Could you check a few things on this model? Use its own coordinates, in mm. Face numbers are marked on the shaded views. A direction names the side the tool comes from. Give positions to 0.01 mm unless a question says otherwise; leave off trailing zeros. Loops run counter-clockwise (first coordinate to the right, second up) from the corner with the lowest first, then second, coordinate; pieces in that order, holes last. Notation, with made-up numbers: M -26,9.5 L 25,9.5 A26 cw 25,36.5 Z; hole C 50.25,63.5 d11. An arc over 180 degrees is marked long. Return JSON: item names as keys, results as strings. Group by question number.
1. If we section it at B-B (z = 83.5): Write out the boundary of the cut face in (x, y).
2. For pin 1 (10 mm diameter, centred on x = 73, y = 48.5, fed in from +Z); pin 2 (8 mm diameter, centred on y = -6, z = 58.5, fed in from +X); pin 3 (5 mm diameter, centred on x = 53, y = 39.5, fed in from -Z); pin 4 (22 mm diameter, centred on x = 213.5, z = -4, fed in from +Y), each with a flat end and sliding along its axis, tell me the tip position at first contact or that it passes through.
3. For the marked faces 1 and 2, which set-ups out of +Z, -Z, +X, -X, +Y, -Y let a thin tool reach every point of the face, with its end or its side?
4. If we mould it in two halves opening along Z, with no side actions, what happens to the marked faces 3, 4 and 5? For each: +Z half, -Z half, draft (parallel to the pull), parting line (faces both ways), or undercut.
5. If we section it at A-A (x = 120): Write out the boundary of the cut face in (y, z).
6. If we section it at C-C (y = 53): Write out the boundary of the cut face in (x, z).
7. If we section it at D-D (x = 59.5): Write out the boundary of the cut face in (y, z).
8. Please list where these lines run through material, in increasing order: line 1 (X direction, y = 59, z = 70); line 2 (Z direction, x = 142.5, y = 12.5); line 3 (Z direction, x = 215, y = 66.05).
```python
from build123d import *

# Parameters (mm, degrees)
SKETCH1_W           = 200
SKETCH1_H           = 125
BOSS_EXTRUDE1_DEPTH = 70
SKETCH2_W           = 210
SKETCH2_H           = 135
BOSS_EXTRUDE2_DEPTH = 10
SKETCH3_R           = 10
BOSS_EXTRUDE5_DEPTH = 5
CUT_EXTRUDE2_DEPTH  = 5
CUT_EXTRUDE3_DEPTH  = 10
SKETCH10_W          = 10
SKETCH10_H          = 125
CUT_EXTRUDE4_DEPTH  = 10
BOSS_EXTRUDE6_DEPTH = 5
SKETCH12_R          = 8
CUT_EXTRUDE5_DEPTH  = 10


with BuildPart() as part:
    # Sketch1 → Boss-Extrude1 (new body)
    with BuildSketch(Plane(origin=(0, 0, 0), x_dir=(1, 0, 0), z_dir=(0, 1, 0))):
        Polygon((210, 0), (0, 0), (0, -135), (5, -135), (210, -135), align=None)
        with Locations((105, -67.5)):
            Rectangle(SKETCH1_W, SKETCH1_H, mode=Mode.SUBTRACT)
    extrude(amount=BOSS_EXTRUDE1_DEPTH)

    # Sketch2 → Boss-Extrude2 (add)
    with BuildSketch(Plane(origin=(0, 0, 0), x_dir=(-1, 0, 0), z_dir=(0, -1, 0))):
        with Locations((-105, -67.5)):
            Rectangle(SKETCH2_W, SKETCH2_H)
    extrude(amount=BOSS_EXTRUDE2_DEPTH)

    # Sketch3 → Boss-Extrude5 (add)
    with BuildSketch(Plane(origin=(0, -10, 0), x_dir=(-1, 0, 0), z_dir=(0, -1, 0))):
        with Locations((-210, 0)):
            Circle(SKETCH3_R)
        Circle(SKETCH3_R)
        with Locations((0, -135)):
            Circle(SKETCH3_R)
        with Locations((-210, -135)):
            Circle(SKETCH3_R)
    extrude(amount=-BOSS_EXTRUDE5_DEPTH)

    # Sketch7 → Cut-Extrude2 (cut)
    with BuildSketch(Plane(origin=(0, -5, 0), x_dir=(1, 0, 0), z_dir=(0, 1, 0))):
        with BuildLine():
            ThreePointArc((215.235533906, -138.535533906), (214.186095741, -136.964938701), (212.333452378, -137.333452378))
            Line((212.333452378, -137.333452378), (214.737615434, -139.737615434))
            ThreePointArc((214.737615434, -139.737615434), (215.106129111, -139.186095741), (215.235533906, -138.535533906))
        make_face()
        with BuildLine():
            Line((214.737615434, -139.737615434), (212.333452378, -137.333452378))
            ThreePointArc((212.333452378, -137.333452378), (212.333452378, -139.737615434), (214.737615434, -139.737615434))
        make_face()
        with BuildLine():
            ThreePointArc((214.737615434, 4.737615434), (212.333452378, 4.737615434), (212.333452378, 2.333452378))
            Line((212.333452378, 2.333452378), (214.737615434, 4.737615434))
        make_face()
        with BuildLine():
            Line((214.737615434, 4.737615434), (212.333452378, 2.333452378))
            ThreePointArc((212.333452378, 2.333452378), (214.186095741, 1.964938701), (215.235533906, 3.535533906))
            ThreePointArc((215.235533906, 3.535533906), (215.106129111, 4.186095741), (214.737615434, 4.737615434))
        make_face()
        with BuildLine():
            ThreePointArc((-4.737615434, 4.737615434), (-4.737615434, 2.333452378), (-2.333452378, 2.333452378))
            Line((-2.333452378, 2.333452378), (-4.737615434, 4.737615434))
        make_face()
        with BuildLine():
            Line((-4.737615434, 4.737615434), (-2.333452378, 2.333452378))
            ThreePointArc((-2.333452378, 2.333452378), (-1.964938701, 2.884972071), (-1.835533906, 3.535533906))
            ThreePointArc((-1.835533906, 3.535533906), (-2.884972071, 5.106129111), (-4.737615434, 4.737615434))
        make_face()
        with BuildLine():
            ThreePointArc((-1.835533906, -138.535533906), (-1.964938701, -137.884972071), (-2.333452378, -137.333452378))
            Line((-2.333452378, -137.333452378), (-4.737615434, -139.737615434))
            ThreePointArc((-4.737615434, -139.737615434), (-2.884972071, -140.106129111), (-1.835533906, -138.535533906))
        make_face()
        with BuildLine():
            Line((-4.737615434, -139.737615434), (-2.333452378, -137.333452378))
            ThreePointArc((-2.333452378, -137.333452378), (-4.737615434, -137.333452378), (-4.737615434, -139.737615434))
        make_face()
    extrude(amount=-CUT_EXTRUDE2_DEPTH, mode=Mode.SUBTRACT)

    # Sketch9 → Cut-Extrude3 (cut)
    with BuildSketch(Plane(origin=(0, 0, 0), x_dir=(1, 0, 0), z_dir=(0, 1, 0))):
        Polygon((195, -130), (200, -125), (205, -120), (205, -15), (200, -10), (195, -5), align=None)
    extrude(amount=-CUT_EXTRUDE3_DEPTH, mode=Mode.SUBTRACT)

    # Sketch10 → Cut-Extrude4 (cut)
    with BuildSketch(Plane(origin=(0, 0, 0), x_dir=(1, 0, 0), z_dir=(0, 1, 0))):
        with Locations((190, -67.5)):
            Rectangle(SKETCH10_W, SKETCH10_H)
    extrude(amount=-CUT_EXTRUDE4_DEPTH, mode=Mode.SUBTRACT)

    # Sketch11 → Boss-Extrude6 (add)
    with BuildSketch(Plane(origin=(0, 70, 0), x_dir=(1, 0, 0), z_dir=(0, 1, 0))):
        with BuildLine():
            ThreePointArc((213.3, -67.5), (215, -65.8), (216.7, -67.5))
            Line((216.7, -67.5), (220, -67.5))
            ThreePointArc((220, -67.5), (217.071067812, -60.428932188), (210, -57.5))
            Line((210, -57.5), (210, -67.5))
            Line((210, -67.5), (213.3, -67.5))
        make_face()
        with BuildLine():
            Line((220, -67.5), (216.7, -67.5))
            ThreePointArc((216.7, -67.5), (215, -69.2), (213.3, -67.5))
            Line((213.3, -67.5), (210, -67.5))
            Line((210, -67.5), (210, -77.5))
            ThreePointArc((210, -77.5), (217.071067812, -74.571067812), (220, -67.5))
        make_face()
        with BuildLine():
            Line((205, -76.160254038), (205, -58.839745962))
            ThreePointArc((205, -58.839745962), (200, -67.5), (205, -76.160254038))
        make_face()
        with BuildLine():
            Line((210, -67.5), (210, -57.5))
            ThreePointArc((210, -57.5), (207.411809549, -57.840741737), (205, -58.839745962))
            Line((205, -58.839745962), (205, -76.160254038))
            ThreePointArc((205, -76.160254038), (207.411809549, -77.159258263), (210, -77.5))
            Line((210, -77.5), (210, -67.5))
        make_face()
        with BuildLine():
            ThreePointArc((10, -67.5), (8.660254038, -62.5), (5, -58.839745962))
            Line((5, -58.839745962), (5, -76.160254038))
            ThreePointArc((5, -76.160254038), (8.660254038, -72.5), (10, -67.5))
        make_face()
        with BuildLine():
            Line((0, -57.5), (0, -67.5))
            Line((0, -67.5), (0, -77.5))
            ThreePointArc((0, -77.5), (2.588190451, -77.159258263), (5, -76.160254038))
            Line((5, -76.160254038), (5, -58.839745962))
            ThreePointArc((5, -58.839745962), (2.588190451, -57.840741737), (0, -57.5))
        make_face()
        with BuildLine():
            Line((0, -77.5), (0, -67.5))
            Line((0, -67.5), (-3.3, -67.5))
            ThreePointArc((-3.3, -67.5), (-5, -69.2), (-6.7, -67.5))
            Line((-6.7, -67.5), (-10, -67.5))
            ThreePointArc((-10, -67.5), (-7.071067812, -74.571067812), (0, -77.5))
        make_face()
        with BuildLine():
            Line((-3.3, -67.5), (0, -67.5))
            Line((0, -67.5), (0, -57.5))
            ThreePointArc((0, -57.5), (-7.071067812, -60.428932188), (-10, -67.5))
            Line((-10, -67.5), (-6.7, -67.5))
            ThreePointArc((-6.7, -67.5), (-5, -65.8), (-3.3, -67.5))
        make_face()
    extrude(amount=-BOSS_EXTRUDE6_DEPTH)

    # Sketch12 → Cut-Extrude5 (cut)
    with BuildSketch(Plane(origin=(0, 0, 0), x_dir=(-1, 0, 0), z_dir=(0, 0, -1))):
        with Locations((-75, 17.5)):
            Circle(SKETCH12_R)
        with Locations((-120, 20)):
            Circle(SKETCH12_R)
    extrude(amount=-CUT_EXTRUDE5_DEPTH, mode=Mode.SUBTRACT)


solid = part.part
```
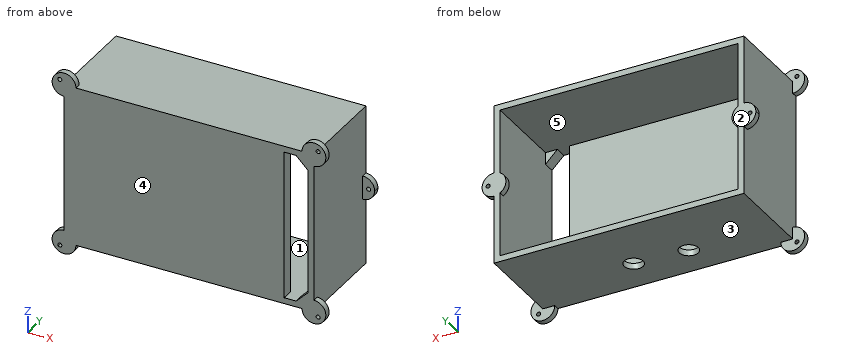
Answer:
{
 "1": {"outline": "M 0,-10 L 185,-10 L 185,0 L 5,0 L 5,70 L 0,70 Z; M 205,-10 L 210,-10 L 210,70 L 205,70 Z"},
 "2": {"pin 1": "stops at z = 135", "pin 2": "stops at x = 210", "pin 3": "stops at z = 0", "pin 4": "stops at y = 70"},
 "3": {"face 1": "+Y", "face 2": "+Z, -Z, +X, -X, +Y"},
 "4": {"face 3": "-Z half", "face 4": "draft", "face 5": "undercut"},
 "5": {"outline": "M -10,0 L 12,0 L 12,5 L 0,5 L 0,130 L 70,130 L 70,135 L -10,135 Z; M 28,0 L 70,0 L 70,5 L 28,5 Z"},
 "6": {"outline": "M 0,0 L 210,0 L 210,135 L 0,135 Z; hole M 5,5 L 205,5 L 205,130 L 5,130 Z"},
 "7": {"outline": "M -10,0 L 70,0 L 70,5 L 0,5 L 0,130 L 70,130 L 70,135 L -10,135 Z"},
 "8": {"line 1": "x = 0 to 5, 205 to 210", "line 2": "z = 0 to 5, 130 to 135", "line 3": "z = 58.84 to 65.8, 69.2 to 76.16"}
}
